Part print with two shaded views. Sizes in mm from the minimum x, y, z corner. A direction names the side the tool comes from. Give positions to 0.01 mm unless a question says otherwise; leave off trailing zeros. Write each loop counter-clockwise with the first axis right and the second up, starting at its lowest first coordinate (ties: lowest second). Pieces come first, ordered by that corner, then holes. Notation, with made-up numbers: (27, 11.5) - (52, 11.5) arc R21 cw to (52, 43.5) - close; hole circle Ø8 at (87.25, 36.25). An arc over 180 degrees is marked (long way). One line per item, written item: value. Start each with the question number.
(1) 3-axis set-ups, long thin cutter, end or side, ignore diameter. For the marked faces 4 and 5: which of +Z, -Z, +X, -X, +Y, -Y reach the whole face in a straight line?
(2) Cut at C-C, the plane z = 19. List the corners of the cut face in (x, y).
(3) Mould opens along X. For the marked faces 1, 2 and 3 say: pulls with the +X half, pulls with the -X half, needs draft (parallel to the pull), parting line crosses it, or undercut.
(4) Cut at D-D, the plane y = 15.5. List the corners of the cut face in (x, z).
(5) Probe L1, parallel to X at y = 10, z = 12.5; L2, parallel to Y at x = 10, z = 1.4. List the from-to ranges inside material, lowest first.
(6) Cut at A-A, the plane y = 10. List the corners of the cut face in (x, z), and give its area (3 significant figures).
(7) Cut at B-B, the plane x = 10. List the corners of the cut face in (y, z).
(8) Drop flat-ended pins along their axis: P1, Ø3, axis at x = 16, y = 10, coming from the +Z side; P2, Ø8, axis at x = 10.5, z = 18.5, coming from the +Y side; P3, Ø10, axis at x = 5, z = 6, coming from the +Y side. Give the stop position or say it passes through.
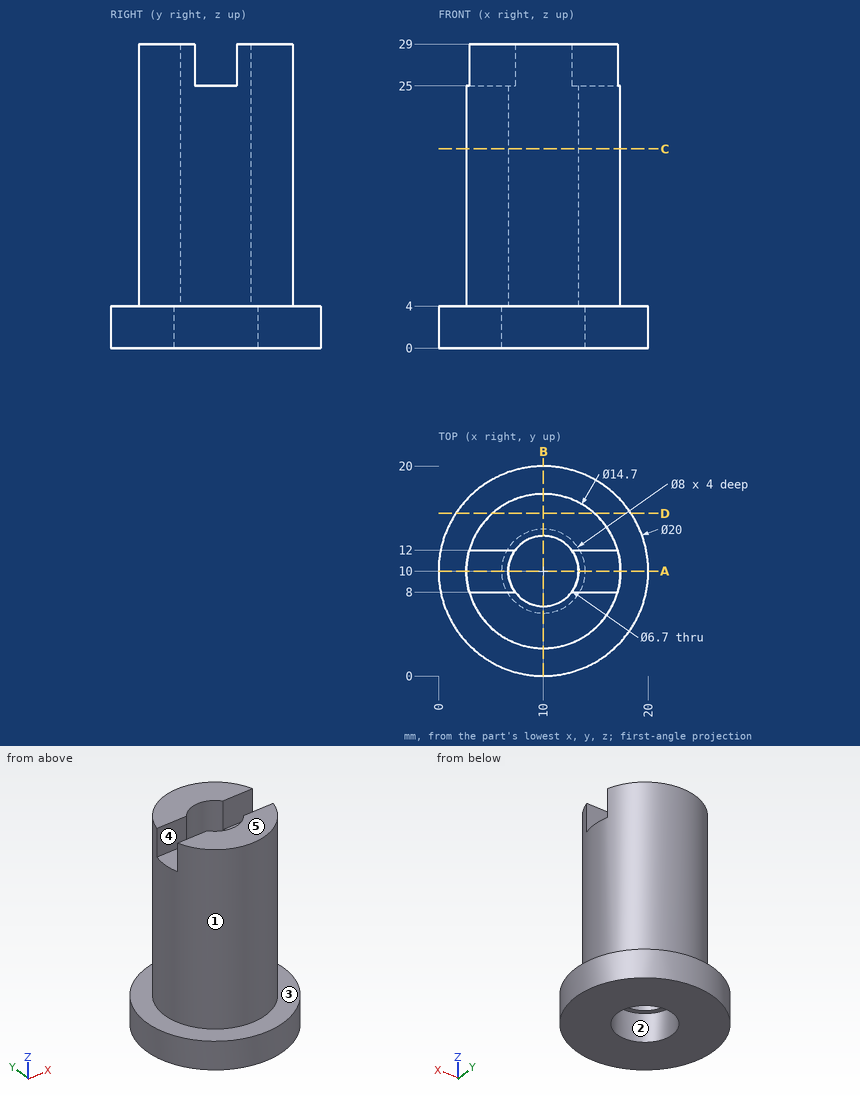
Answers follow:
1. face 4: +Z, +X, -X
1. face 5: +Z, +X, -X, +Y, -Y
2. outline: circle Ø14.7 at (10, 10); hole circle Ø6.7 at (10, 10)
3. face 1: parting line crosses it
3. face 2: undercut
3. face 3: needs draft
4. outline: (1.65, 0) - (18.35, 0) - (18.35, 4) - (14.88, 4) - (14.88, 29) - (5.12, 29) - (5.12, 4) - (1.65, 4) - close
5. L1: x = 2.65 to 6.65, 13.35 to 17.35
5. L2: y = 0 to 6, 14 to 20
6. outline: (0, 0) - (6, 0) - (6, 4) - (6.65, 4) - (6.65, 25) - (2.65, 25) - (2.65, 4) - (0, 4) - close; (13.35, 4) - (14, 4) - (14, 0) - (20, 0) - (20, 4) - (17.35, 4) - (17.35, 25) - (13.35, 25) - close
6. area: 216 mm²
7. outline: (0, 0) - (6, 0) - (6, 4) - (6.65, 4) - (6.65, 29) - (2.65, 29) - (2.65, 4) - (0, 4) - close; (13.35, 4) - (14, 4) - (14, 0) - (20, 0) - (20, 4) - (17.35, 4) - (17.35, 29) - (13.35, 29) - close
8. P1: stops at z = 25
8. P2: stops at y = 17.35
8. P3: stops at y = 19.99
